Check sheet for the modelled part. Datum: model origin and axes. Units: mm. A direction names the side the tool comes from. Give positions to 0.01 mm unless a question says otherwise; leave off trailing zeros. Write each loop counter-clockwise with the first axis right and the second up, starting at its lowest first coordinate (ties: lowest second). Pieces come first, ordered by that corner, then holes. Notation, with made-up numbers: (-12, 71) -> (46, 71) arc R35 cw to (46, 103) -> close; hole circle Ø8 at (-31.5, 56). An arc over 180 degrees is marked (long way). Return JSON: item names as keys, results as strings.
from build123d import *

# Parameters (mm, degrees)
PAD008_DEPTH    = 1
PAD009_DEPTH    = 13.1
POCKET001_DEPTH = 1


with BuildPart() as part:
    # Sketch012 → Pad008 (new body)
    with BuildSketch(Plane.XY):
        with BuildLine():
            ThreePointArc((-2.828427, 4.6), (-4.713465, 2.635004), (-5.4, 0))
            ThreePointArc((-5.4, 0), (-4.713465, -2.635004), (-2.828427, -4.6))
            Line((0, -4.6), (-2.828427, -4.6))
            Line((0, -4.6), (2.828427, -4.6))
            ThreePointArc((2.828427, -4.6), (4.713465, -2.635004), (5.4, 0))
            ThreePointArc((5.4, 0), (4.713465, 2.635004), (2.828427, 4.6))
            Line((0, 4.6), (2.828427, 4.6))
            Line((0, 4.6), (-2.828427, 4.6))
        make_face()
    extrude(amount=PAD008_DEPTH)

    # Sketch013 → Pad009 (join)
    with BuildSketch(Plane.XY):
        with BuildLine():
            ThreePointArc((-2.828427, 4.6), (-4.713465, 2.635004), (-5.4, 0))
            ThreePointArc((-5.4, 0), (-4.713465, -2.635004), (-2.828427, -4.6))
            Line((0, -4.6), (-2.828427, -4.6))
            Line((0, -4.6), (2.828427, -4.6))
            ThreePointArc((2.828427, -4.6), (4.713465, -2.635004), (5.4, 0))
            ThreePointArc((5.4, 0), (4.713465, 2.635004), (2.828427, 4.6))
            Line((0, 4.6), (2.828427, 4.6))
            Line((0, 4.6), (-2.828427, 4.6))
        make_face()
    extrude(amount=-PAD009_DEPTH)

    # Sketch014 → Revolution002 (revolve)
    with BuildSketch(Plane.YZ):
        Polygon((0, 1), (0, 3), (5.9, 3), (6.9, 1), align=None)
    revolve(axis=Axis((0, 0, 0), (0, 0, 1)))

    # Sketch015 (on Face1 of Revolution002) → Pocket001 (cut)
    with BuildSketch(Plane.XY.offset(3)):
        with BuildLine():
            ThreePointArc((-3.315, 1.28), (-4.595, 0), (-3.315, -1.28))
            Line((-3.315, -1.28), (3.315, -1.28))
            ThreePointArc((3.315, -1.28), (4.595, 0), (3.315, 1.28))
            Line((-3.315, 1.28), (3.315, 1.28))
        make_face()
    extrude(amount=-POCKET001_DEPTH, mode=Mode.SUBTRACT)


solid = part.part
(1) Cross-section at A-A on x = 0. Enter the section's corners in (y, z).
Reply:
{"outline": "(-6.9, 1) -> (-4.6, 1) -> (-4.6, -13.1) -> (4.6, -13.1) -> (4.6, 1) -> (6.9, 1) -> (5.9, 3) -> (1.28, 3) -> (1.28, 2) -> (-1.28, 2) -> (-1.28, 3) -> (-5.9, 3) -> close"}
(2) Thickness scan on L1, parallel to Y at x = -2.5, z = -2.5; L2, parallel to Z at x = 0.25, y = -5.5; L3, parallel to Y at x = 0, z = 1.5. Record the ranges inside material, lowest first.
Reply:
{"L1": "-4.6 to 4.6", "L2": "1 to 3", "L3": "-6.65 to 6.65"}
(3) Set-up check for faces 1 (the flat face through (0, -4.6, -6)), 2 (the flat face through (-1, -5, 1)), 3 (the flat face through (0, -3, 3)), 4 (the cylindrical face through (-4.595, 0.028, 2.507)): record each of +Z, -Z, +X, -X, +Y, -Y from which the full face is reachable in a straight line by a thin tool's end or side.
Reply:
{"face 1": "-Z, +X, -X, -Y", "face 2": "-Z", "face 3": "+Z, +X, -X, +Y, -Y", "face 4": "+Z"}
(4) Depth check by flat-ended pin: pin 1 Ø3 at (y, z) = (1, -10) entering from -X; pin 2 Ø5 at (x, z) = (4, -11.5) entering from +Y; pin 3 Ø1.7 at (x, z) = (-0.5, -8.5) entering from -Y. Enter the tip coordinate at first touch or a pass-through.
Reply:
{"pin 1": "x = -5.4", "pin 2": "y = 4.6", "pin 3": "y = -4.6"}
(5) Release check for a two-part mould opening along Y. For faces 5 (the flat face through (0, 4.6, -6)), 6 (the flat face through (0, 0, -13.1)), 7 (the cylindrical face through (4.595, -0.028, 2.507)), 8 (the flat face through (0, -1.28, 2.5)) record: pulls with the +Y half, pulls with the -Y half, needs draft (parallel to the pull), parting line crosses it, or undercut.
Reply:
{"face 5": "pulls with the +Y half", "face 6": "needs draft", "face 7": "undercut", "face 8": "undercut"}
(6) Cross-section at B-B on z = -1. Enter the section's corners in (x, y), then the cut area to 3 significant figures.
Reply:
{"outline": "(-5.4, 0) arc R5.4 ccw to (-2.83, -4.6) -> (2.83, -4.6) arc R5.4 ccw to (5.4, 0) arc R5.4 ccw to (2.83, 4.6) -> (-2.83, 4.6) arc R5.4 ccw to start", "area": "85.5 mm^2"}
